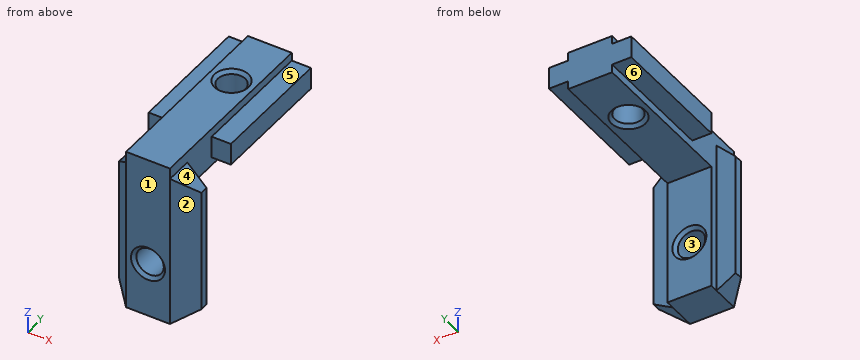
```python
from build123d import *

# Parameters (mm, degrees)
EXTRUDE_1_DEPTH     = 30
SKETCH_2_W          = 7
SKETCH_2_H          = 35
EXTRUDE_2_DEPTH     = 4
CUT_EXTRUDE_1_DEPTH = 6
SKETCH_4_W          = 15
SKETCH_4_H          = 4
EXTRUDE_3_DEPTH     = 23


with BuildPart() as part:
    # Эскиз1 → Бобышка-Вытянуть1 (new body)
    with BuildSketch(Plane.XY):
        Polygon((4, 0), (-4, 0), (-4, -1.5), (-7.5, -1.5), (-7.5, -3), (-4, -6.5), (4, -6.5), (7.5, -3), (7.5, -1.5), (4, -1.5), align=None)
    extrude(amount=EXTRUDE_1_DEPTH)

    # Эскиз2 → Бобышка-Вытянуть2 (add, symmetric)
    with BuildSketch(Plane(origin=(0, 0, 0), x_dir=(0, 0, -1), z_dir=(1, 0, 0))):
        with Locations((-26.5, 11)):
            Rectangle(SKETCH_2_W, SKETCH_2_H)
    extrude(amount=EXTRUDE_2_DEPTH, both=True)

    # Эскиз3 → Вырез-Вытянуть1 (cut, through all)
    with BuildSketch(Plane(origin=(0, -1.5, 0), x_dir=(1, 0, 0), z_dir=(0, 1, 0))):
        Polygon((-4, 0), (-7.5, -2.020725942), (-7.5, 0), align=None)
        Polygon((-4, -28), (-7.5, -24.5), (-7.5, -30), (-4, -30), align=None)
        Polygon((4, -30), (4, -28), (7.5, -24.5), (7.5, -30), align=None)
        Polygon((7.5, 0), (4, 0), (7.5, -2.020725942), align=None)
    extrude(amount=-CUT_EXTRUDE_1_DEPTH, mode=Mode.SUBTRACT)

    # Эскиз4 → Бобышка-Вытянуть3 (add)
    with BuildSketch(Plane(origin=(0, 28.5, 0), x_dir=(1, 0, 0), z_dir=(0, 1, 0))):
        with Locations((0, -26.5)):
            Rectangle(SKETCH_4_W, SKETCH_4_H)
    extrude(amount=-EXTRUDE_3_DEPTH)

    # Эскиз6 → Отверстие обработанное метчиком M61 (revolve, cut)
    with BuildSketch(Plane(origin=(0, -6.5, 10), x_dir=(0, 0, -1), z_dir=(1, 0, 0))):
        Polygon((0, 0), (0, 6.5), (3.1, 6.5), (2.5, 5.9), (2.5, 0.6), (3.1, 0), align=None)
    revolve(axis=Axis((0, -12.85, 10), (0, 1, 0)), mode=Mode.SUBTRACT)

    # Эскиз8 → Отверстие обработанное метчиком M62 (revolve, cut)
    with BuildSketch(Plane(origin=(0, 17.5, 30), x_dir=(0, -1, 0), z_dir=(1, 0, 0))):
        Polygon((0, 0), (0, 7), (3.1, 7), (2.5, 6.4), (2.5, 0.6), (3.1, 0), align=None)
    revolve(axis=Axis((0, 17.5, 36.35), (0, 0, -1)), mode=Mode.SUBTRACT)


solid = part.part
```
Model file for the job. Use its own axes, mm. Face numbers are marked on the shaded views. A direction names the side the tool comes from. Coordinates: 2 decimals unless noted, no trailing zeros. Order: outer loops, then holes, each group sorted by start corner. A loop starts at its lowest first (then second) coordinate and runs counter-clockwise, first axis right, second up. Notation, with made-up numbers: (-17.5, -37) - (-8.5, -37) arc R19 ccw to (-8.5, -6) - close; hole circle Ø1 at (48.5, -38.75). An arc over 180 degrees is marked (long way). Return JSON: item names as keys, results as strings. Group by question number.
1) Saw through at C-C, the plane y = 17.5. Write the cut outline in (x, z).
2) Saw through at B-B, the plane x = 0. Write the cut outline in (y, z), plus the area to 3 significant figures.
3) Mould opens along X. For the marked faces 1, 2 and 3 say: released by +X, released by -X, zero draft, split by the parting line, or undercut.
4) Tool access for the marked faces 4, 5 and 6: list every direction of +Z, -Z, +X, -X, +Y, -Y with a clear straight run to the whole face (end or side of a thin tool).
5) Saw through at D-D, the plane z = 3.5. Write the cut outline in (x, y).
6) Flat gauge pins, fed straight in: P1, Ø1.8, axis at x = 5.5, z = 9.5, coming from the +Y side; P2, Ø8, axis at x = 4.5, y = 21.5, coming from the -Z side; P3, Ø3, axis at x = -5, z = 26.5, coming from the -Y side; P4, Ø4, axis at x = 6.5, z = 26, coming from the -Y side. Where does each tip first touch, or does it go through?
7) Probe line 1 (X direction, y = -2.85, z = 10); line 2 (Z direction, x = 0, y = -4.75); line 3 (Y direction, x = 0, z = 26.85). List the from-to ranges inside material, lowest first. Write a range as from..to.
8) Saw through at A-A, the plane z = 10. Write the cut outline in (x, y).
Values found:
{
 "1": {"outline": "(-7.5, 24.5) - (-4, 24.5) - (-4, 23) - (-3.1, 23) - (-2.5, 23.6) - (-2.5, 29.4) - (-3.1, 30) - (-4, 30) - (-4, 28.5) - (-7.5, 28.5) - close; (2.5, 23.6) - (3.1, 23) - (4, 23) - (4, 24.5) - (7.5, 24.5) - (7.5, 28.5) - (4, 28.5) - (4, 30) - (3.1, 30) - (2.5, 29.4) - close"},
 "2": {"outline": "(-6.5, 0) - (0, 0) - (0, 6.9) - (-0.6, 7.5) - (-5.9, 7.5) - (-6.5, 6.9) - close; (-6.5, 13.1) - (-5.9, 12.5) - (-0.6, 12.5) - (0, 13.1) - (0, 23) - (14.4, 23) - (15, 23.6) - (15, 29.4) - (14.4, 30) - (-6.5, 30) - close; (20, 23.6) - (20.6, 23) - (28.5, 23) - (28.5, 30) - (20.6, 30) - (20, 29.4) - close", "area": "326 mm²"},
 "3": {"face 1": "zero draft", "face 2": "released by +X", "face 3": "undercut"},
 "4": {"face 4": "+Z, +X, -Y", "face 5": "+Z, +X, +Y, -Y", "face 6": "-Z, -X, +Y"},
 "5": {"outline": "(-7.5, -3) - (-4, -6.5) - (4, -6.5) - (7.5, -3) - (7.5, -1.5) - (4, -1.5) - (4, 0) - (-4, 0) - (-4, -1.5) - (-7.5, -1.5) - close"},
 "6": {"P1": "stops at y = -1.5", "P2": "stops at z = 23", "P3": "stops at y = -6.5", "P4": "stops at y = -6"},
 "7": {"line 1": "x = -7.5..-2.5, 2.5..7.5", "line 2": "z = 0..7.5, 12.5..30", "line 3": "y = -6.5..15, 20..28.5"},
 "8": {"outline": "(-7.5, -3) - (-4, -6.5) - (-3.1, -6.5) - (-2.5, -5.9) - (-2.5, -0.6) - (-3.1, 0) - (-4, 0) - (-4, -1.5) - (-7.5, -1.5) - close; (2.5, -5.9) - (3.1, -6.5) - (4, -6.5) - (7.5, -3) - (7.5, -1.5) - (4, -1.5) - (4, 0) - (3.1, 0) - (2.5, -0.6) - close"}
}
